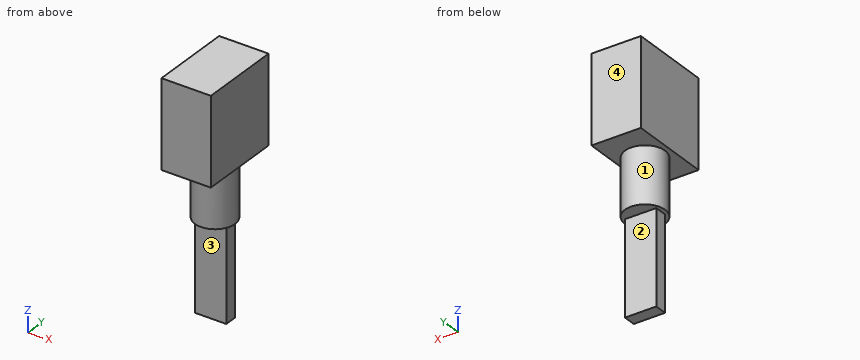
```python
from build123d import *

# Parameters (mm, degrees)
SKETCH_1_W      = 7.9
SKETCH_1_H      = 13.2
EXTRUDE_1_DEPTH = 14
SKETCH_2_R      = 3.2
EXTRUDE_2_DEPTH = 9
SKETCH_3_W      = 5
SKETCH_3_H      = 2
EXTRUDE_3_DEPTH = 15


with BuildPart() as part:
    # 草圖1 → 填料-伸長1 (new body)
    with BuildSketch(Plane.XY):
        with Locations((-28.615519845, -65.707444045)):
            Rectangle(SKETCH_1_W, SKETCH_1_H)
    extrude(amount=EXTRUDE_1_DEPTH)

    # 草圖2 → 填料-伸長2 (add)
    with BuildSketch(Plane(origin=(0, 0, 0), x_dir=(-1, 0, 0), z_dir=(0, 0, -1))):
        with Locations((28.615519845, -65.707444045)):
            Circle(SKETCH_2_R)
    extrude(amount=EXTRUDE_2_DEPTH)

    # 草圖3 → 填料-伸長3 (add)
    with BuildSketch(Plane(origin=(0, 0, -9), x_dir=(-1, 0, 0), z_dir=(0, 0, -1))):
        with Locations((28.615519845, -65.707444045)):
            Rectangle(SKETCH_3_W, SKETCH_3_H)
    extrude(amount=EXTRUDE_3_DEPTH)


solid = part.part
```
Check sheet for the modelled part. Datum: model origin and axes. Units: mm. Face numbers are marked on the shaded views. A direction names the side the tool comes from. Round coordinates to 2 decimals unless told otherwise and drop trailing zeros. Order: outer loops, then holes, each group sorted by start corner. A loop starts at its lowest first (then second) coordinate and runs counter-clockwise, first axis right, second up. Notation, with made-up numbers: M 70,73 L 129,73 A9 ccw 129,82 Z; hole C -20,42 d1. An arc over 180 degrees is marked long. Answer in a Markdown table with one row per item.
(1) Section check D-D on x = -30.25. Record the boundary of the cut face in (y, z).
Findings:
| item | result |
|---|---|
| outline | M -72.31,0 L -68.46,0 L -68.46,-9 L -66.71,-9 L -66.71,-24 L -64.71,-24 L -64.71,-9 L -62.96,-9 L -62.96,0 L -59.11,0 L -59.11,14 L -72.31,14 Z |
(2) Set-up check for the marked faces 1, 2, 3 and 4: record each of +Z, -Z, +X, -X, +Y, -Y from which the full face is reachable in a straight line by a thin tool's end or side.
Findings:
| item | result |
|---|---|
| face 1 | -Z |
| face 2 | -Z, +X, -X, +Y |
| face 3 | -Z, +X, -X, -Y |
| face 4 | +Z, -Z, +X, -X, +Y |
(3) Section check B-B on y = -63.5. Record the boundary of the cut face in (x, z), plus the area to 3 significant figures.
Findings:
| item | result |
|---|---|
| outline | M -32.57,0 L -30.93,0 L -30.93,-9 L -26.3,-9 L -26.3,0 L -24.67,0 L -24.67,14 L -32.57,14 Z |
| area | 152 mm^2 |
(4) Section check A-A on x = -28. Record the boundary of the cut face in (y, z).
Findings:
| item | result |
|---|---|
| outline | M -72.31,0 L -68.85,0 L -68.85,-9 L -66.71,-9 L -66.71,-24 L -64.71,-24 L -64.71,-9 L -62.57,-9 L -62.57,0 L -59.11,0 L -59.11,14 L -72.31,14 Z |
(5) Material ranges on line 1 along Z through (x, y) = (-26, -63); line 2 along Y through (x, z) = (-30, -18); line 3 along Z through (x, y) = (-31.25, -64.25), recorded low to high. Write a range as from..to.
Findings:
| item | result |
|---|---|
| line 1 | z = 0..14 |
| line 2 | y = -66.71..-64.71 |
| line 3 | z = -9..14 |
(6) Section check C-C on z = -10. Record the boundary of the cut face in (x, y).
Findings:
| item | result |
|---|---|
| outline | M -31.12,-66.71 L -26.12,-66.71 L -26.12,-64.71 L -31.12,-64.71 Z |
(7) Gauge pin test, flat ends, axial feed: pin 1 (0.6 mm diameter, centred on y = -65.5, z = -18, fed in from -X); pin 2 (0.6 mm diameter, centred on y = -66, z = -15, fed in from +X); pin 3 (2.5 mm diameter, centred on x = -29, z = -15.5, fed in from +Y). Record the tip position at first contact, or that the pin passes through.
Findings:
| item | result |
|---|---|
| pin 1 | stops at x = -31.12 |
| pin 2 | stops at x = -26.12 |
| pin 3 | stops at y = -64.71 |
